The model under review builds one solid part; all positions refer to its coordinate system, in mm. Face numbers are marked on the shaded views. Give positions to 0.01 mm unless a question says otherwise; leave off trailing zeros. Loops run counter-clockwise (first coordinate to the right, second up) from the corner with the lowest first, then second, coordinate; pieces in that order, holes last. Notation, with made-up numbers: (31.5, -24) - (82.5, -24) arc R20 ccw to (82.5, -9) - close; hole circle Ø9 at (-13.5, 88.5). An arc over 180 degrees is marked (long way). Answer as a JSON object with one key per item and string values.
from build123d import *

# Parameters (mm, degrees)
F1_DEPTH = 6
F0_R     = 1
F2_DEPTH = 2.5
F3_R     = 4
F4_DEPTH = 2
F5_R     = 2
F6_DEPTH = 1
F7_R     = 0.25
F8_DEPTH = 5
F9_R     = 1


with BuildPart() as f1:
    # F0 (on Top) → F1 (new body)
    with BuildSketch(Plane.XY):
        with BuildLine():
            ThreePointArc((14.3325547763, -4.4246890947), (14.8322001342, -2.2373732764), (15, 0))
            ThreePointArc((15, 0), (14.8322001342, 2.2373732764), (14.3325547763, 4.4246890947))
            ThreePointArc((14.3325547763, 4.4246890947), (9.6924552433, 11.447982851), (2, 14.8660687473))
            ThreePointArc((2, 14.8660687473), (0, 15), (-2, 14.8660687473))
            ThreePointArc((-2, 14.8660687473), (-9.6924552433, 11.447982851), (-14.3325547763, 4.4246890947))
            ThreePointArc((-14.3325547763, 4.4246890947), (-14.8322001342, 2.2373732764), (-15, 0))
            ThreePointArc((-15, 0), (-14.8322001342, -2.2373732764), (-14.3325547763, -4.4246890947))
            ThreePointArc((-14.3325547763, -4.4246890947), (0, -15), (14.3325547763, -4.4246890947))
        make_face()
    extrude(amount=F1_DEPTH)

    # F0 (on Top) → F2 (join)
    with BuildSketch(Plane.XY):
        with BuildLine():
            ThreePointArc((-18.6370210525, 2.2264732485), (-16.1947323323, 2.132199877), (-15, 0))
            ThreePointArc((-15, 0), (-14.8322001342, 2.2373732764), (-14.3325547763, 4.4246890947))
            Line((-14.3325547763, 4.4246890947), (-18.6370210525, 2.2264732485))
        make_face()
        with BuildLine():
            ThreePointArc((-18.6370210525, -2.2264732485), (-16.1947323323, -2.132199877), (-15, 0))
            ThreePointArc((-15, 0), (-16.1947323323, 2.132199877), (-18.6370210525, 2.2264732485))
            ThreePointArc((-18.6370210525, 2.2264732485), (-20, 0), (-18.6370210525, -2.2264732485))
        make_face()
        with Locations((-17.5, 0)):
            Circle(F0_R, mode=Mode.SUBTRACT)
        with BuildLine():
            ThreePointArc((14.3325547763, 4.4246890947), (14.8322001342, 2.2373732764), (15, 0))
            ThreePointArc((15, 0), (16.1947323323, 2.132199877), (18.6370210525, 2.2264732485))
            Line((18.6370210525, 2.2264732485), (14.3325547763, 4.4246890947))
        make_face()
        with BuildLine():
            ThreePointArc((18.6370210525, 2.2264732485), (16.1947323323, 2.132199877), (15, 0))
            ThreePointArc((15, 0), (16.1947323323, -2.132199877), (18.6370210525, -2.2264732485))
            ThreePointArc((18.6370210525, -2.2264732485), (19.632199877, -1.3052676677), (20, 0))
            ThreePointArc((20, 0), (19.632199877, 1.3052676677), (18.6370210525, 2.2264732485))
        make_face()
        with Locations((17.5, 0)):
            Circle(F0_R, mode=Mode.SUBTRACT)
        with BuildLine():
            ThreePointArc((18.6370210525, -2.2264732485), (16.1947323323, -2.132199877), (15, 0))
            ThreePointArc((15, 0), (14.8322001342, -2.2373732764), (14.3325547763, -4.4246890947))
            Line((14.3325547763, -4.4246890947), (18.6370210525, -2.2264732485))
        make_face()
        with BuildLine():
            Line((-18.6370210525, -2.2264732485), (-14.3325547763, -4.4246890947))
            ThreePointArc((-14.3325547763, -4.4246890947), (-14.8322001342, -2.2373732764), (-15, 0))
            ThreePointArc((-15, 0), (-16.1947323323, -2.132199877), (-18.6370210525, -2.2264732485))
        make_face()
    extrude(amount=F2_DEPTH)

    # F3 (on face) → F4 (cut)
    with BuildSketch(Plane.XY.offset(6)):
        Circle(F3_R)
    extrude(amount=-F4_DEPTH, mode=Mode.SUBTRACT)

    # F5
    f5_edges = [f1.edges().sort_by_distance(p)[0] for p in [
        (15, 0, 6),
    ]]
    fillet(f5_edges, radius=F5_R)

    # F0 (on Top) → F6 (join)
    with BuildSketch(Plane.XY):
        with BuildLine():
            ThreePointArc((-2, 14.8660687473), (0, 15), (2, 14.8660687473))
            Line((2, 14.8660687473), (2, 15.0660687473))
            Line((2, 15.0660687473), (0, 15.0660687473))
            Line((0, 15.0660687473), (-2, 15.0660687473))
            Line((-2, 15.0660687473), (-2, 14.8660687473))
        make_face()
    extrude(amount=F6_DEPTH)

    # F7 (on face) → F8 (join)
    with BuildSketch(Plane(origin=(0, 15.0660687473, 0), x_dir=(-1, 0, 0), z_dir=(0, 1, 0))):
        with Locations((-0.8499287069, 0.4951201845)):
            Circle(F7_R)
        with Locations((0.8499287069, 0.4951201845)):
            Circle(F7_R)
    extrude(amount=F8_DEPTH)

    # F9
    f9_edges = [f1.edges().sort_by_distance(p)[0] for p in [
        (16.484788, -3.325581, 2.5),
        (-16.484788, 3.325581, 2.5),
        (-4, 0, 6),
    ]]
    fillet(f9_edges, radius=F9_R)


solid = f1.part
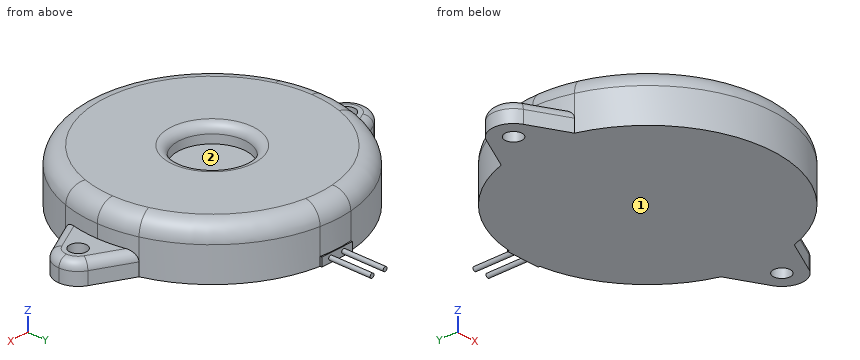
Q1. The part is to be moulded in two halves that separate along X. For the marked faces 1 and 2, say which applies: +X half, -X half, draft (parallel to the pull), parting line (faces both ways), or undercut.
Results:
{"face 1": "draft", "face 2": "undercut"}
Q2. Consider section B-B, the plane x = 0. State the section outline as (y, z) points, plus the area to 3 significant figures.
Results:
{"outline": "(-15, 0) - (15.07, 0) - (15.07, 1) - (15, 1) - (15, 4) arc R2 ccw to (13, 6) - (5, 6) arc R1 ccw to (4, 5) - (4, 4) - (-4, 4) - (-4, 5) arc R1 ccw to (-5, 6) - (-13, 6) arc R2 ccw to (-15, 4) - close", "area": "162 mm^2"}
Q3. To check wall thickness, follow probe 1 along X at (y, z) = (-7.5, 3.65); probe 2 along X at (y, z) = (-1, 4.85); probe 3 along Z at (x, y) = (2, 4.5). State the ranges of each line that lie inside material, in increasing order. Write a range as [from, to].
Results:
{"probe 1": "x = [-12.99, 12.99]", "probe 2": "x = [-14.78, -3.87], [3.87, 14.78]", "probe 3": "z = [0, 6]"}
Q4. Consider section A-A, the plane z = 3.3. State the section outline as (x, y) points.
Results:
{"outline": "circle Ø30 at (0, 0)"}
Q5. Clearance check with flat-ended pins moving along their axes: pin 1 Ø5 at (x, y) = (-16, 1.5) entering from +Z; pin 2 Ø2.5 at (x, y) = (1.5, -1.5) entering from +Z; pin 3 Ø2.5 at (x, y) = (-17.5, 0) entering from +Z. State where each tip first meets the part, or that it passes through.
Results:
{"pin 1": "stops at z = 5.92", "pin 2": "stops at z = 4", "pin 3": "stops at z = 2.5"}
